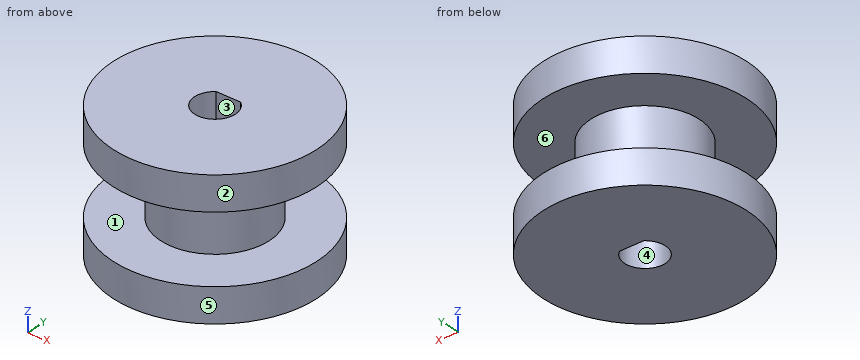
```python
from build123d import *

# Parameters (mm, degrees)
ESQUISSE1_R        = 15
ESQUISSE1_R_2      = 3
BOSS_EXTRU_2_DEPTH = 5
ESQUISSE3_R        = 8
ESQUISSE3_R_2      = 3
BOSS_EXTRU_3_DEPTH = 10
ESQUISSE4_R        = 15
ESQUISSE4_R_2      = 3
BOSS_EXTRU_4_DEPTH = 5
BOSS_EXTRU_5_DEPTH = 20


with BuildPart() as part:
    # Esquisse1 → Boss.-Extru.2 (new body)
    with BuildSketch(Plane.XY):
        Circle(ESQUISSE1_R)
        Circle(ESQUISSE1_R_2, mode=Mode.SUBTRACT)
    extrude(amount=BOSS_EXTRU_2_DEPTH)

    # Esquisse3 → Boss.-Extru.3 (add)
    with BuildSketch(Plane.XY.offset(5)):
        Circle(ESQUISSE3_R)
        Circle(ESQUISSE3_R_2, mode=Mode.SUBTRACT)
    extrude(amount=BOSS_EXTRU_3_DEPTH)

    # Esquisse4 → Boss.-Extru.4 (add)
    with BuildSketch(Plane.XY.offset(15)):
        Circle(ESQUISSE4_R)
        Circle(ESQUISSE4_R_2, mode=Mode.SUBTRACT)
    extrude(amount=BOSS_EXTRU_4_DEPTH)

    # Esquisse1_4 → Boss.-Extru.5 (add)
    with BuildSketch(Plane.XY):
        with BuildLine():
            ThreePointArc((1.8, 2.4), (0, 3), (-1.8, 2.4))
            Line((-1.8, 2.4), (1.8, 2.4))
        make_face()
    extrude(amount=BOSS_EXTRU_5_DEPTH)


solid = part.part
```
Part model, mm, in its own coordinate system. Face numbers are marked on the shaded views. A direction names the side the tool comes from. Round coordinates to 2 decimals unless told otherwise and drop trailing zeros. Loops run counter-clockwise (first coordinate to the right, second up) from the corner with the lowest first, then second, coordinate; pieces in that order, holes last. Notation, with made-up numbers: (57.25, -12) -> (78.25, -12) arc R25 ccw to (78.25, 18) -> close; hole circle Ø4 at (-23.5, -23). An arc over 180 degrees is marked (long way). Use CSV: the item, a comma, the result in double quotes. Start each with the question number.
1) Cut at B-B, the plane x = 0. Write the cut outline in (y, z).
2) Wall check: L1, parallel to Y at x = 0, z = 13.5; L2, parallel to Z at x = -12.5, y = -2.25; L3, parallel to Y at x = 2.5, z = 6.25. Give the ranges that are in metal, low to high. Write a range as [from, to].
3) Cut at C-C, the plane z = 8. Write the cut outline in (x, y), plus the area to 3 significant figures.
4) Drop flat-ended pins along their axis: P1, Ø8, axis at x = 2, y = 1, coming from the +Z side; P2, Ø2, axis at x = 1, z = 9, coming from the -Y side; P3, Ø3, axis at y = 11.5, z = 4.5, coming from the +X side; P4, Ø1, axis at y = -11, z = 16.5, coming from the +X side. Give the stop position or say it passes through.
5) Cut at A-A, the plane y = 0. Write the cut outline in (x, z).
6) Which spindle directions (+Z, -Z, +X, -X, +Y, -Y) get a long thin tool onto all of the face, cutting with end or side? Do the marked faces 1 and 2. Say none if no direction does.
7) Pull direction Y, two halves, no side cores. Call the marked faces 3, 4, 5 and 6: +Y half, -Y half, draft (parallel to the pull), parting line (faces both ways), or undercut.
8) Cut at D-D, the plane y = 9.5. Write the cut outline in (x, z), plus the area to 3 significant figures.
Determined:
1,outline,"(-15, 0) -> (-3, 0) -> (-3, 20) -> (-15, 20) -> (-15, 15) -> (-8, 15) -> (-8, 5) -> (-15, 5) -> close; (2.4, 0) -> (15, 0) -> (15, 5) -> (8, 5) -> (8, 15) -> (15, 15) -> (15, 20) -> (2.4, 20) -> close"
2,L1,"y = [-8, -3], [2.4, 8]"
2,L2,"z = [0, 5], [15, 20]"
2,L3,"y = [-7.6, -1.66], [1.66, 7.6]"
3,outline,"circle Ø16 at (0, 0); hole (-1.8, 2.4) arc R3 ccw (long way) to (1.8, 2.4) -> close"
3,area,"174 mm2"
4,P1,"stops at z = 20"
4,P2,"stops at y = -8"
4,P3,"stops at x = 11.18"
4,P4,"stops at x = 10.71"
5,outline,"(-15, 0) -> (-3, 0) -> (-3, 20) -> (-15, 20) -> (-15, 15) -> (-8, 15) -> (-8, 5) -> (-15, 5) -> close; (3, 0) -> (15, 0) -> (15, 5) -> (8, 5) -> (8, 15) -> (15, 15) -> (15, 20) -> (3, 20) -> close"
6,face 1,"none"
6,face 2,"+Z, -Z"
7,face 3,"undercut"
7,face 4,"undercut"
7,face 5,"parting line"
7,face 6,"draft"
8,outline,"(-11.61, 0) -> (11.61, 0) -> (11.61, 5) -> (-11.61, 5) -> close; (-11.61, 15) -> (11.61, 15) -> (11.61, 20) -> (-11.61, 20) -> close"
8,area,"232 mm2"
